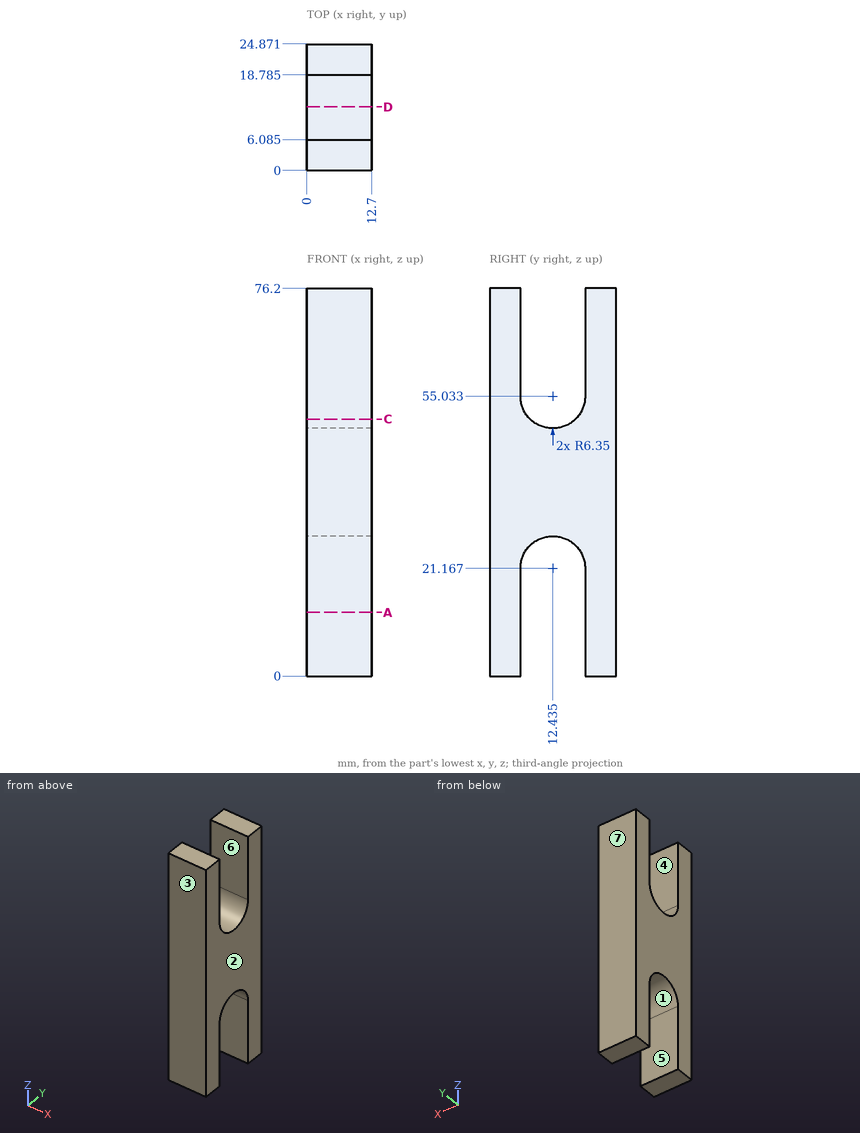
Study the drawing (mm; zero at the part's minimum x, y, z) and answer. A direction names the side the tool comes from. Coordinates: 2 decimals unless noted, no trailing zeros. Write each loop counter-clockwise with the first axis right and the second up, starting at its lowest first coordinate (ties: lowest second). Pieces come first, ordered by that corner, then holes. Notation, with made-up numbers: (35, 7.25) - (94, 7.25) arc R24 ccw to (94, 30.25) - close; hole circle Ø1 at (7.5, 70.5). An arc over 180 degrees is marked (long way). Return JSON: item names as keys, results as strings. Group by question number.
1. A cutting plane is placed at D-D, the plane y = 12.5. Determine the outline of the cut face in (x, z), plus the area to 3 significant figures.
2. Straight lines are drawn through the part: L1, parallel to Y at x = 3.25, z = 21 (1 decimal); L2, parallel to Z at x = 4, y = 12; L3, parallel to Z at x = 8, y = 7. For each, find the intervals that lie inside material, in ascending order.
3. Determine the mould class of the marked faces 1, 2, 3 and 4 for opening direction Y: released by +Y, released by -Y, zero draft, split by the parting line, or undercut.
4. A cutting plane is placed at A-A, the plane z = 12.5. Determine the outline of the cut face in (x, y) (1 decimal).
5. Which of the six approach directions +Z, -Z, +X, -X, +Y, -Y give full straight-line access (tool end or side, diameter ignored) to the marked faces 5, 6 and 7?
6. A cutting plane is placed at C-C, the plane z = 50.5. Determine the outline of the cut face in (x, y).
Ans:
{
 "1": {"outline": "(0, 27.52) - (12.7, 27.52) - (12.7, 48.68) - (0, 48.68) - close", "area": "269 mm²"},
 "2": {"L1": "0 to 6.1, 18.8 to 24.9", "L2": "27.5 to 48.7", "L3": "24.45 to 51.75"},
 "3": {"face 1": "undercut", "face 2": "zero draft", "face 3": "released by -Y", "face 4": "undercut"},
 "4": {"outline": "(0, 0) - (12.7, 0) - (12.7, 6.1) - (0, 6.1) - close; (0, 18.8) - (12.7, 18.8) - (12.7, 24.9) - (0, 24.9) - close"},
 "5": {"face 5": "-Z, +X, -X", "face 6": "+Z, +X, -X", "face 7": "+Z, -Z, +X, -X, +Y"},
 "6": {"outline": "(0, 0) - (12.7, 0) - (12.7, 7.99) - (0, 7.99) - close; (0, 16.88) - (12.7, 16.88) - (12.7, 24.87) - (0, 24.87) - close"}
}
